```python
from build123d import *

# Parameters (mm, degrees)
F3_START = -2
F3_DEPTH = 23
F4_DEPTH = 25
F5_DEPTH = 1.5
F6_SIZE  = 1
F7_SIZE2 = 0.7
F7_SIZE  = 2
F8_SIZE  = 0.2
F9_DEPTH = 25
F10_W    = 4.5
F10_H    = 5.8


with BuildPart() as f1:
    # F0 (on Front) → F1 (revolve)
    with BuildSketch(Plane.XZ):
        Polygon((-4.9, 9), (-4.9, 0), (0, 0), (0, 19), (-0.7, 19), (-0.7, 10), (-4.9, 10), align=None)
    revolve(axis=Axis((0, 0, 9.5), (0, 0, -1)))

    # F2 (on Front) → F3 (cut)
    with BuildSketch(Plane.XZ.offset(F3_START)):
        with BuildLine():
            Line((1.5, 0), (1.5, 8.1))
            ThreePointArc((1.5, 8.1), (0, 9.6), (-1.5, 8.1))
            Line((-1.5, 8.1), (-1.5, 0))
            Line((-1.5, 0), (1.5, 0))
        make_face()
    extrude(amount=-F3_DEPTH, mode=Mode.SUBTRACT)

    # F2 (on Front) → F4 (cut)
    with BuildSketch(Plane.XZ):
        with BuildLine():
            Line((1.5, 0), (1.5, 8.1))
            ThreePointArc((1.5, 8.1), (0, 9.6), (-1.5, 8.1))
            Line((-1.5, 8.1), (-1.5, 0))
            Line((-1.5, 0), (1.5, 0))
        make_face()
    extrude(amount=-F4_DEPTH, mode=Mode.SUBTRACT)

    # F1_face (on face) → F5 (join)
    with BuildSketch(Plane(origin=(0, -0.5723183731, 0), x_dir=(1, 0, 0), z_dir=(0, 0, -1))):
        with BuildLine():
            Line((1.5, -0.5723183731), (1.5, -5.237079889))
            ThreePointArc((1.5, -5.237079889), (2.8861739379, 3.3874796015), (-4.9, -0.5723183731))
            ThreePointArc((-4.9, -0.5723183731), (-3.9597979746, -3.458492311), (-1.5, -5.237079889))
            Line((-1.5, -5.237079889), (-1.5, -0.5723183731))
            Line((-1.5, -0.5723183731), (1.5, -0.5723183731))
        make_face()
    extrude(amount=F5_DEPTH)

    # F6
    f6_edges = [f1.edges().sort_by_distance(p)[0] for p in [
        (-4.9, 0, 4.25),
        (2.886174, -3.959798, -1.5),
        (-3.959798, 2.886174, -1.5),
    ]]
    chamfer(f6_edges, length=F6_SIZE)

    # F7
    f7_edges = [f1.edges().sort_by_distance(p)[0] for p in [
        (0.7, 0, 19),
    ]]
    f7_side = f1.faces().sort_by_distance((0.7, 0, 14.5))[0]
    chamfer(f7_edges, length=F7_SIZE, length2=F7_SIZE2, reference=f7_side)

    # F8
    f8_edges = [f1.edges().sort_by_distance(p)[0] for p in [
        (4.9, 0, 10),
    ]]
    chamfer(f8_edges, length=F8_SIZE)

    # F5_face (on face) → F9 (cut)
    with BuildSketch(Plane(origin=(0, 0, 3.8942483753), x_dir=(-1, 0, 0), z_dir=(0, 1, 0))):
        with BuildLine():
            ThreePointArc((1.5, 4.2057516247), (0, 5.7057516247), (-1.5, 4.2057516247))
            Line((-1.5, 4.2057516247), (-1.5, -5.3942483753))
            Line((-1.5, -5.3942483753), (1.5, -5.3942483753))
            Line((1.5, -5.3942483753), (1.5, 4.2057516247))
        make_face()
    extrude(amount=-F9_DEPTH, mode=Mode.SUBTRACT)

    # F10 (on face) → F11 (join, up to the next surface of F1)
    with BuildSketch(Plane(origin=(0, 0, -1.5), x_dir=(1, 0, 0), z_dir=(0, 0, -1))):
        Rectangle(F10_W, F10_H)
    extrude(until=Until.NEXT, dir=(0, 0, 1))


solid = f1.part
```
The listing builds one solid part. Answer for the finished solid, in the listing's coordinates (mm). A direction names the side the tool comes from. Give positions to 0.01 mm unless a question says otherwise; leave off trailing zeros. Write each loop counter-clockwise with the first axis right and the second up, starting at its lowest first coordinate (ties: lowest second). Pieces come first, ordered by that corner, then holes. Notation, with made-up numbers: (-5.5, -22.5) -> (40.5, -22.5) arc R18 cw to (40.5, -0.5) -> close; hole circle Ø5 at (6, -4). An arc over 180 degrees is marked (long way). Use one line per item in the form item = value.
1) Straight lines are drawn through the part: probe 1 along Z at (x, y) = (2.5, -1.5); probe 2 along Y at (x, z) = (1.25, 0); probe 3 along X at (y, z) = (-3.5, 5). For each, find the intervals that lie inside material, in ascending order.
Result:
probe_1 = -1.5 to 10
probe_2 = -2.9 to 2.9
probe_3 = -3.43 to -1.5, 1.5 to 3.43
2) For a pull along X with two mould halves and no side action, classify faces 4 (the cylindrical face through (0.7, 0, 13.5)), 5 (the flat face through (0, 0, -1.5)), 6 (the flat face through (0, -2.9, 4)) as +X half, -X half, draft (parallel to the pull), parting line (faces both ways), or undercut.
Result:
face_4 = parting line
face_5 = draft
face_6 = undercut
3) Section A-A on z = 0.5 is taken. Write down the section's boundary in (x, y), plus the area to 3 significant figures.
Result:
outline = (-1.5, -4.66) -> (-1.5, -2.9) -> (1.5, -2.9) -> (1.5, -4.66) arc R4.9 ccw to (1.5, 4.66) -> (1.5, 2.9) -> (-1.5, 2.9) -> (-1.5, 4.66) arc R4.9 ccw to start
area = 63.9 mm²
4) Section B-B on z = 11.25 is taken. Write down the section's boundary in (x, y).
Result:
outline = circle Ø1.4 at (0, 0)
5) Section C-C on z = 17.5 is taken. Write down the section's boundary in (x, y) (3 decimals).
Result:
outline = circle Ø1.05 at (0, 0)
6) A tool of negligible diameter and unlimited length cuts with its end or side. For faces 1 (the conical face through (0.274, -0.21, 18.014)), 2 (the cylindrical face through (0, -3.9, 9.6)), 3 (the flat face through (1.5, 4, 3)), from which of +Z, -Z, +X, -X, +Y, -Y can it reach the whole face along a straight path? Write none if from no direction.
Result:
face_1 = +Z
face_2 = -Z, -Y
face_3 = -Z, +Y
7) Each of these flat-tipped pins is pushed along its axis until it touches: P1, Ø2, axis at y = -2, z = 3, coming from the +X side; P2, Ø1.4, axis at y = 4, z = 2.5, coming from the -X side; P3, Ø1.5, axis at x = -1.5, z = 12, coming from the +Y side; P4, Ø1.4, axis at y = -4, z = 1, coming from the +X side. Where does it stop, or does it pass through?
Result:
P1 = 4.8
P2 = -3.62
P3 = through
P4 = 3.62
